```python
from build123d import *

# Parameters (mm, degrees)
EXTRUDE_1_DEPTH     = 270
SKETCH_2_R          = 1.5
CUT_EXTRUDE_1_DEPTH = 1


with BuildPart() as part:
    # Эскиз1 → Бобышка-Вытянуть1 (new body)
    with BuildSketch(Plane(origin=(0, 0, 0), x_dir=(0, 0, -1), z_dir=(1, 0, 0))):
        Polygon((-5, 5), (-4, 5), (-4, -4), (5, -4), (5, -5), (-5, -5), align=None)
    extrude(amount=EXTRUDE_1_DEPTH)

    # Эскиз2 → Вырез-Вытянуть1 (cut)
    with BuildSketch(Plane(origin=(0, -4, 0), x_dir=(1, 0, 0), z_dir=(0, 1, 0))):
        with Locations(Location((135, 0.5, 0), (0, 0, 270))):
            Circle(SKETCH_2_R)
        with Locations(Location((72.5, 0.5, 0), (0, 0, 270))):
            Circle(SKETCH_2_R)
        with Locations(Location((10, 0.5, 0), (0, 0, 270))):
            Circle(SKETCH_2_R)
        with Locations(Location((260, 0.5, 0), (0, 0, 270))):
            Circle(SKETCH_2_R)
        with Locations(Location((197.5, 0.5, 0), (0, 0, 270))):
            Circle(SKETCH_2_R)
    extrude(amount=-CUT_EXTRUDE_1_DEPTH, mode=Mode.SUBTRACT)


solid = part.part
```
Can you work these out from the model? Positions are in its coordinate system, mm. A direction names the side the tool comes from. Coordinates: 2 decimals unless noted, no trailing zeros. Write each loop counter-clockwise with the first axis right and the second up, starting at its lowest first coordinate (ties: lowest second). Pieces come first, ordered by that corner, then holes. Notation, with made-up numbers: M 49,52.5 L 74,52.5 A17 cw 74,68.5 Z; hole C 22,81.25 d6. An arc over 180 degrees is marked long. Answer as CSV lines item,"result".
Item 1: Imagine slicing it at C-C on y = 3. List the corners of the cut face in (x, z) for me.
Geometry results:
outline,"M 0,4 L 270,4 L 270,5 L 0,5 Z"
Item 2: Please list where these lines run through material, in increasing order: line 1 along X through (y, z) = (-4.5, -0.5); line 2 along Z through (x, y) = (197.5, -4.35); line 3 along Y through (x, z) = (162, -1.75).
Geometry results:
line 1,"x = 0 to 8.5, 11.5 to 71, 74 to 133.5, 136.5 to 196, 199 to 258.5, 261.5 to 270"
line 2,"z = -5 to -2, 1 to 5"
line 3,"y = -5 to -4"
Item 3: Imagine slicing it at A-A on z = -0.5. List the corners of the cut face in (x, y) for me, plus the area to 3 significant figures.
Geometry results:
outline,"M 0,-5 L 8.5,-5 L 8.5,-4 L 0,-4 Z; M 11.5,-5 L 71,-5 L 71,-4 L 11.5,-4 Z; M 74,-5 L 133.5,-5 L 133.5,-4 L 74,-4 Z; M 136.5,-5 L 196,-5 L 196,-4 L 136.5,-4 Z; M 199,-5 L 258.5,-5 L 258.5,-4 L 199,-4 Z; M 261.5,-5 L 270,-5 L 270,-4 L 261.5,-4 Z"
area,"255 mm2"
Item 4: I'm going to push flat-ended pins straight in: P1, Ø5, axis at x = 10, z = -0.5, coming from the -Y side; P2, Ø1, axis at x = 132.5, y = 3.5, coming from the -Z side; P3, Ø2, axis at x = 161.5, z = -4, coming from the +Y side. Where does each tip first touch, or does it pass through?
Geometry results:
P1,"stops at y = -5"
P2,"stops at z = 4"
P3,"stops at y = -4"
Item 5: We'd pull the mould along X, two halves only. Please class faces 1 (the flat face through (0, -4.4, 2.2)), 2 (the flat face through (270, -4.4, 2.2)), 3 (the flat face through (133, 1, 4)): +X half, -X half, draft (parallel to the pull), parting line (faces both ways), or undercut.
Geometry results:
face 1,"-X half"
face 2,"+X half"
face 3,"draft"
Item 6: On a 3-axis mill with a long thin cutter (end or side, diameter ignored), from which of +Z, -Z, +X, -X, +Y, -Y can I reach the whole of each face in a straight line? I mean faces 4 (the flat face through (133, -4, 0)), 5 (the flat face through (133, -5, 0)). Say none if no direction works.
Geometry results:
face 4,"-Z, +X, -X, +Y"
face 5,"+Z, -Z, +X, -X, -Y"
Item 7: Imagine slicing it at B-B on x = 110.5. List the corners of the cut face in (y, z) for me, plus the area to 3 significant figures.
Geometry results:
outline,"M -5,-5 L -4,-5 L -4,4 L 5,4 L 5,5 L -5,5 Z"
area,"19.0 mm2"
